from build123d import *

# Parameters (mm, degrees)
SKETCH1_W           = 152.4
SKETCH1_H           = 63.5
BOSS_EXTRUDE1_DEPTH = 101.6
SKETCH3_W           = 146.05
SKETCH3_H           = 95.34
CUT_EXTRUDE1_DEPTH  = 6.35


with BuildPart() as part:
    # Sketch1 → Boss-Extrude1 (new body)
    with BuildSketch(Plane.XY):
        Rectangle(SKETCH1_W, SKETCH1_H)
    extrude(amount=-BOSS_EXTRUDE1_DEPTH)

    # Sketch3 → Cut-Extrude1 (cut)
    with BuildSketch(Plane(origin=(0, 31.75, 0), x_dir=(1, 0, 0), z_dir=(0, 1, 0))):
        with Locations((0, 50.8)):
            Rectangle(SKETCH3_W, SKETCH3_H)
    cut_extrude1 = extrude(amount=-CUT_EXTRUDE1_DEPTH, mode=Mode.SUBTRACT)

    # Mirror1: Cut-Extrude1 across plane
    add(cut_extrude1.mirror(Plane.ZX), mode=Mode.SUBTRACT)


solid = part.part
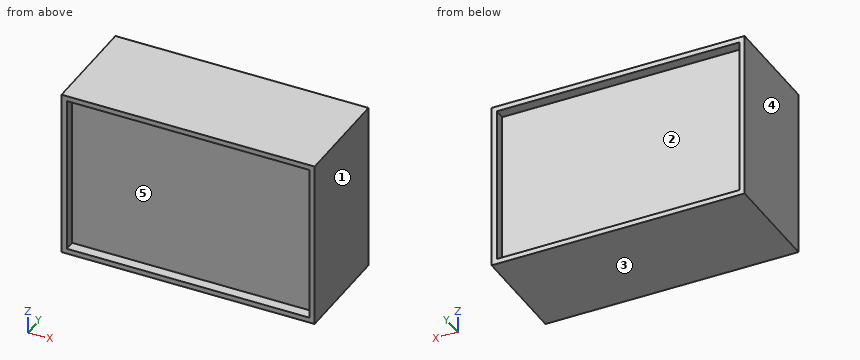
Could you check a few things on this model? Use its own coordinates, in mm. Face numbers are marked on the shaded views. A direction names the side the tool comes from. Give positions to 0.01 mm unless a question says otherwise; leave off trailing zeros. Order: outer loops, then holes, each group sorted by start corner. A loop starts at its lowest first (then second) coordinate and runs counter-clockwise, first axis right, second up.
1. Suppose I cut it at B-B (z = -34). Write out the boundary of the cut face in (x, y) (3 decimals), plus the area to 3 significant figures.
Answers below:
outline: (-76.2, -31.75) - (-73.025, -31.75) - (-73.025, -25.4) - (73.025, -25.4) - (73.025, -31.75) - (76.2, -31.75) - (76.2, 31.75) - (73.025, 31.75) - (73.025, 25.4) - (-73.025, 25.4) - (-73.025, 31.75) - (-76.2, 31.75) - close
area: 7,820 mm2
2. Thinking about a two-plate mould opening in X: for the marked faces 1, 2 and 3, which applies, +X half, -X half, draft (parallel to the pull), parting line (faces both ways), or undercut?
Answers below:
face 1: +X half
face 2: undercut
face 3: draft
3. I need wall thicknesses on L1, parallel to Z at x = -49.5, y = 25.5; L2, parallel to X at y = -27, z = -83 (3 decimals); L3, parallel to Y at x = 27, z = -52. Which ranges of each line are inside material? Lowest first, please.
Answers below:
L1: z = -101.6 to -98.47, -3.13 to 0
L2: x = -76.2 to -73.025, 73.025 to 76.2
L3: y = -25.4 to 25.4
4. Which directions (+Z, -Z, +X, -X, +Y, -Y) give clear straight access to the entire face, cutting with the end or side of a thin tool? Please do the marked faces 4 and 5.
Answers below:
face 4: +Z, -Z, -X, +Y, -Y
face 5: -Y
5. Suppose I cut it at A-A (x = 28.5). Write out the boundary of the cut face in (y, z), plus the area to 3 significant figures.
Answers below:
outline: (-31.75, -101.6) - (31.75, -101.6) - (31.75, -98.47) - (25.4, -98.47) - (25.4, -3.13) - (31.75, -3.13) - (31.75, 0) - (-31.75, 0) - (-31.75, -3.13) - (-25.4, -3.13) - (-25.4, -98.47) - (-31.75, -98.47) - close
area: 5,240 mm2
6. For pin 1 (8 mm diameter, centred on x = -22, z = -36, fed in from -Y); pin 2 (1.5 mm diameter, centred on x = -51, z = -19.5, fed in from +Y), each with a flat end and sliding along its axis, tell me the tip position at first contact or that it passes through.
Answers below:
pin 1: stops at y = -25.4
pin 2: stops at y = 25.4
